For this review, take the finished solid that the model builds, in its own axes (mm). A direction names the side the tool comes from. Give positions to 0.01 mm unless a question says otherwise; leave off trailing zeros. Write each loop counter-clockwise with the first axis right and the second up, starting at its lowest first coordinate (ties: lowest second). Pieces come first, ordered by that corner, then holes.
1) We need section D-D on x = 50. Give the boundary of the cut face in (y, z).
2) Machinability: for faces 4 (the face through (0, -297, -62)), 5 (the face through (-70, -289, -35)), 6 (the face through (64.94, -286.91, -65.16)), which of the approach directions +Z, -Z, +X, -X, +Y, -Y give a long, thin tool a straight path to every point of the face, cutting with its end or side? Answer none if there is none.
3) Draft analysis for pull direction Y (two halves, no side actions). For faces 1 (the face through (-10, -197, -3)), 2 (the face through (40, -171.719, -3)), 3 (the face through (45.754, -206.532, -2.958)), state which applies: pulls with the +Y half, pulls with the -Y half, needs draft (parallel to the pull), parting line crosses it, or undercut.
4) We need section A-A on y = -213. Give the boundary of the cut face in (x, z), and give its area (3 significant figures).
5) We need section C-C on z = -90. Give the boundary of the cut face in (x, y).
6) Wall thickness on line 1 along X through (y, z) = (-285, -7); line 2 along Z through (x, y) = (35, -287); line 3 along Y through (x, z) = (-50, -3.25): over which ranges is each line inside the solid? List them lowest first.
7) For P1, Ø5, axis at x = -12.5, y = -229.5, coming from the -Z side; P2, Ø15, axis at y = -254.5, z = -18.5, coming from the -X side; P3, Ø5, axis at y = -265, z = -15.5, coming from the +X side, all flat-tipped, find the tip position at first contact; note any pin that passes through.
8) We need section B-B on x = 0. Give the boundary of the cut face in (y, z), and give its area (3 significant figures).
from build123d import *

# Parameters (mm, degrees)
F0_R     = 4.25
F1_DEPTH = 6
F3_DEPTH = 120
F5_DEPTH = 120
F7_REACH = 132.1169232427
F9_DEPTH = 300.001


with BuildPart() as f1:
    # F0 (on Top) → F1 (new body)
    with BuildSketch(Plane.XY):
        with BuildLine():
            Line((-70, -171.7190429163), (-70, -291.7190429163))
            ThreePointArc((-70, -291.7190429163), (0, -300), (70, -291.7190429163))
            Line((70, -291.7190429163), (70, -171.7190429163))
            Line((70, -171.7190429163), (10, -171.7190429163))
            Line((10, -171.7190429163), (10, -221.7190429163))
            Line((10, -221.7190429163), (0, -221.7190429163))
            Line((0, -221.7190429163), (-10, -221.7190429163))
            Line((-10, -221.7190429163), (-10, -171.7190429163))
            Line((-10, -171.7190429163), (-70, -171.7190429163))
        make_face()
        with Locations((-50, -206.7190429163)):
            Circle(F0_R, mode=Mode.SUBTRACT)
        with Locations((50, -206.7190429163)):
            Circle(F0_R, mode=Mode.SUBTRACT)
    extrude(amount=-F1_DEPTH)

    # F2 (on face) → F3 (join)
    with BuildSketch(Plane(origin=(0, 0, -6), x_dir=(1, 0, 0), z_dir=(0, 0, -1))):
        with BuildLine():
            Line((-54, 237.9850195496), (-54, 289.1701427966))
            ThreePointArc((-54, 289.1701427966), (-57.0030799982, 288.5931744788), (-60, 287.9850195496))
            Line((-60, 287.9850195496), (-60, 237.9850195496))
            Line((-60, 237.9850195496), (-54, 237.9850195496))
        make_face()
        with BuildLine():
            ThreePointArc((60, 287.9850195496), (65.0098735772, 286.8956043973), (70, 285.7190429163))
            Line((70, 285.7190429163), (70, 291.7190429163))
            ThreePointArc((70, 291.7190429163), (0, 300), (-70, 291.7190429163))
            Line((-70, 291.7190429163), (-70, 285.7190429163))
            ThreePointArc((-70, 285.7190429163), (-65.0098735772, 286.8956043973), (-60, 287.9850195496))
            ThreePointArc((-60, 287.9850195496), (-57.0030799982, 288.5931744788), (-54, 289.1701427966))
            ThreePointArc((-54, 289.1701427966), (0, 294.1689505794), (54, 289.1701427966))
            ThreePointArc((54, 289.1701427966), (57.0030799982, 288.5931744788), (60, 287.9850195496))
        make_face()
        with BuildLine():
            Line((60, 237.9850195496), (60, 287.9850195496))
            ThreePointArc((60, 287.9850195496), (57.0030799982, 288.5931744788), (54, 289.1701427966))
            Line((54, 289.1701427966), (54, 237.9850195496))
            Line((54, 237.9850195496), (60, 237.9850195496))
        make_face()
    extrude(amount=F3_DEPTH)

    # F4 (on face) → F5 (cut, through all)
    with BuildSketch(Plane.YZ.offset(60)):
        Polygon((-237.9850195496, -126), (-237.9850195496, -6), (-287.9850195496, -56), (-287.9850195496, -126), align=None)
    extrude(amount=-F5_DEPTH, mode=Mode.SUBTRACT)

    f7_end = Plane(origin=(57, -262.9850195496, -31), x_dir=(0, 0.7071067812, 0.7071067812), z_dir=(0, 0.7071067812, -0.7071067812))
    # F6 (on face) → F7 (cut, up to a plane its end follows)
    with BuildSketch(Plane(origin=(0, 0, -126), x_dir=(1, 0, 0), z_dir=(0, 0, -1))):
        Polygon((-54, 287.9850195496), (-54, 289.1701427966), (-60, 287.9850195496), align=None)
        Polygon((60, 287.9850195496), (54, 289.1701427966), (54, 287.9850195496), align=None)
    f7_long = extrude(amount=-F7_REACH, mode=Mode.PRIVATE)
    add(split(f7_long, bisect_by=f7_end, keep=Keep.TOP, mode=Mode.PRIVATE), mode=Mode.SUBTRACT)

    # F8 (on Front) → F9 (cut, through all)
    with BuildSketch(Plane.XZ):
        with BuildLine():
            Line((8, -84), (0, -84))
            Line((0, -84), (-8, -84))
            ThreePointArc((-8, -84), (-14, -90), (-8, -96))
            Line((-8, -96), (0, -96))
            Line((0, -96), (8, -96))
            ThreePointArc((8, -96), (14, -90), (8, -84))
        make_face()
        with BuildLine():
            Line((6, -48), (6, -40))
            ThreePointArc((6, -40), (0, -34), (-6, -40))
            Line((-6, -40), (-6, -48))
            Line((-6, -48), (-6, -56))
            ThreePointArc((-6, -56), (0, -62), (6, -56))
            Line((6, -56), (6, -48))
        make_face()
    extrude(amount=F9_DEPTH, mode=Mode.SUBTRACT)


solid = f1.part
Results list:
1. outline: (-295.8, -126) - (-289.89, -126) - (-289.89, -6) - (-210.97, -6) - (-210.97, 0) - (-295.8, 0) - close; (-202.47, -6) - (-171.72, -6) - (-171.72, 0) - (-202.47, 0) - close
2. face 4: +Y, -Y
2. face 5: +Z, -Z, -X, +Y, -Y
2. face 6: -Z, +Y
3. face 1: needs draft
3. face 2: pulls with the +Y half
3. face 3: undercut
4. outline: (-70, -6) - (-10, -6) - (-10, 0) - (-70, 0) - close; (10, -6) - (70, -6) - (70, 0) - (10, 0) - close
4. area: 720 mm2
5. outline: (-70, -291.72) arc R300 ccw to (-14, -299.67) - (-14, -293.84) arc R294.17 cw to (-54, -289.17) - (-60, -287.99) arc R294.17 cw to (-70, -285.72) - close; (14, -299.67) arc R300 ccw to (70, -291.72) - (70, -285.72) arc R294.17 cw to (60, -287.99) - (54, -289.17) arc R294.17 cw to (14, -293.84) - close
6. line 1: x = -60 to -54, 54 to 60
6. line 2: z = -6 to 0
6. line 3: y = -295.8 to -210.97, -202.47 to -171.72
7. P1: stops at z = -6
7. P2: stops at x = -60
7. P3: stops at x = 60
8. outline: (-300, -126) - (-294.17, -126) - (-294.17, -96) - (-300, -96) - close; (-300, -84) - (-294.17, -84) - (-294.17, -62) - (-300, -62) - close; (-300, -34) - (-294.17, -34) - (-294.17, -6) - (-221.72, -6) - (-221.72, 0) - (-300, 0) - close
8. area: 936 mm2
